Can you work these out from the drawing? Everything is in mm from the part's minimum corner. Coordinates: 2 decimals unless noted, no trailing zeros. Write each loop counter-clockwise with the first axis right and the second up, starting at its lowest first coordinate (ties: lowest second). Pieces come first, ordered by that corner, then holes.
(1) Imagine slicing it at A-A, the plane z = 34. List the corners of the cut face in (x, y) for me, plus the area to 3 significant figures.
(2) For pin 1 Ø3 at (y, z) = (6, 22) entering from -X; pin 2 Ø2 at (y, z) = (6.5, 33.5) entering from -X; pin 3 Ø3 at (x, y) = (3.9, 3.9) entering from -Z, each with a flat end and sliding along its axis, tell me the tip position at first contact or that it passes through.
(3) Imagine slicing it at B-B, the plane x = 0.5. List the corners of the cut face in (y, z) for me.
(4) Thinking about a two-plate mould opening in X: for the marked faces 1 and 2, which applies, released by +X, released by -X, zero draft, split by the parting line, or undercut?
(5) Please list where these lines run through material, in increasing order: probe 1 along X at (y, z) = (3.9, 9.5); probe 2 along X at (y, z) = (3.9, 24.25).
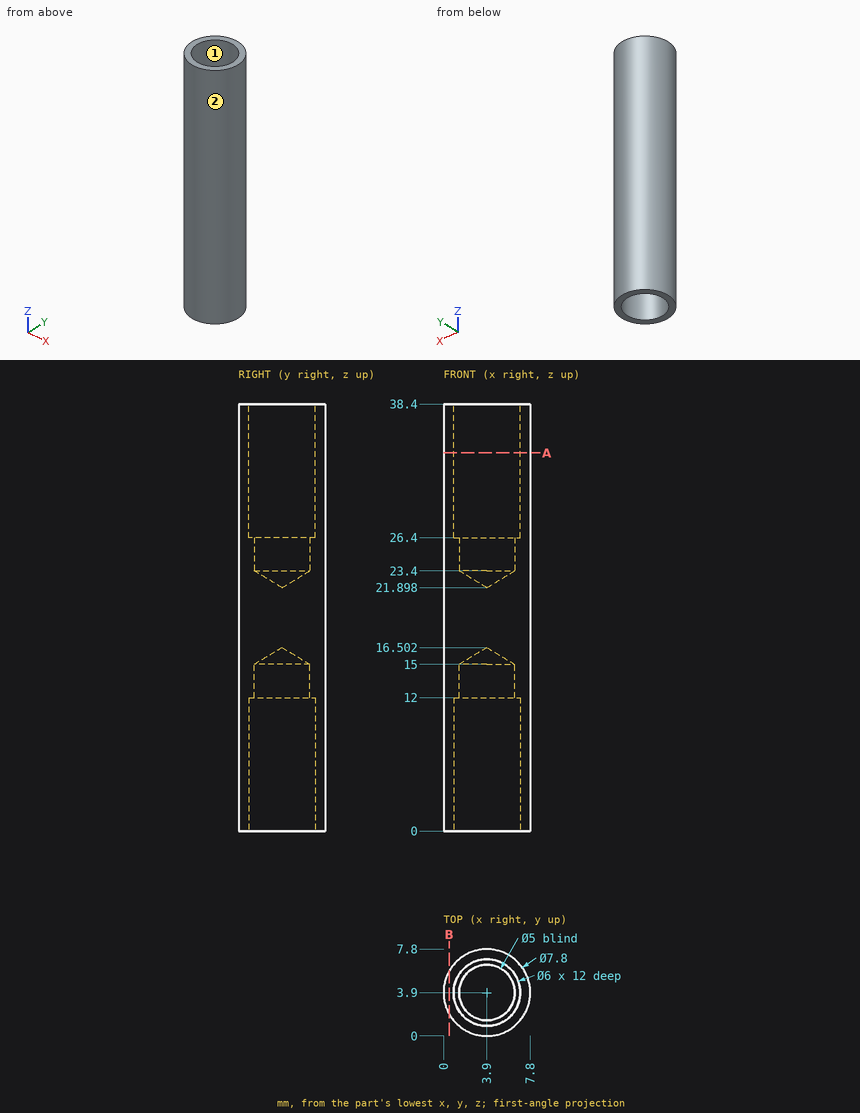
Recorded:
1. outline: circle Ø7.8 at (3.9, 3.9); hole circle Ø6 at (3.9, 3.9)
1. area: 19.5 mm2
2. pin 1: stops at x = 0.05
2. pin 2: stops at x = 0.34
2. pin 3: stops at z = 15.6
3. outline: (1.99, 0) - (5.81, 0) - (5.81, 38.4) - (1.99, 38.4) - close
4. face 1: undercut
4. face 2: split by the parting line
5. probe 1: x = 0 to 0.9, 6.9 to 7.8
5. probe 2: x = 0 to 1.4, 6.4 to 7.8
